CAD build for the part. Positions are in the model's coordinates, mm. A direction names the side the tool comes from. Round coordinates to 2 decimals unless told otherwise and drop trailing zeros. Loops run counter-clockwise (first coordinate to the right, second up) from the corner with the lowest first, then second, coordinate; pieces in that order, holes last.
from build123d import *

# Parameters (mm, degrees)
F1_DEPTH = 12.7
F2_R     = 6.35
F3_DEPTH = 76.201
F4_R     = 6.35
F5_DEPTH = 12.7


with BuildPart() as f1:
    # F0 (on Top) → F1 (new body, symmetric)
    with BuildSketch(Plane.XY):
        Polygon((12.7, -38.1), (12.7, 0), (12.7, 38.1), (-12.7, 38.1), (-12.7, 12.7), (-38.1, 12.7), (-38.1, 0), (-38.1, -12.7), (-12.7, -12.7), (-12.7, -38.1), align=None)
    extrude(amount=F1_DEPTH, both=True)

    # F2 (on face) → F3 (cut, through all)
    with BuildSketch(Plane(origin=(0, 38.1, 0), x_dir=(-1, 0, 0), z_dir=(0, 1, 0))):
        Circle(F2_R)
    extrude(amount=-F3_DEPTH, mode=Mode.SUBTRACT)

    # F4 (on face) → F5 (cut)
    with BuildSketch(Plane(origin=(-38.1, 0, 0), x_dir=(0, -1, 0), z_dir=(-1, 0, 0))):
        Circle(F4_R)
    extrude(amount=-F5_DEPTH, mode=Mode.SUBTRACT)


solid = f1.part
Item 1: Cut at C-C (y = 0). List the corners of the cut face in (x, z), plus the area to 3 significant figures.
Verdict:
outline: (-38.1, -12.7) - (12.7, -12.7) - (12.7, 12.7) - (-38.1, 12.7) - (-38.1, 6.35) - (-25.4, 6.35) - (-25.4, -6.35) - (-38.1, -6.35) - close; hole circle Ø12.7 at (0, 0)
area: 1,000 mm2
Item 2: Mould opens along Y. For faces 4 (the cylindrical face through (1.38, 0.53, -6.2)), 5 (the flat face through (3, 38.1, 6)), 6 (the flat face through (-25.4, 0, 0)) say: released by +Y, released by -Y, zero draft, split by the parting line, or undercut.
Verdict:
face 4: zero draft
face 5: released by +Y
face 6: undercut
Item 3: Wall check: L1, parallel to Z at x = -31.5, y = 0; L2, parallel to X at y = -28, z = -9.25; L3, parallel to X at y = 30.5, z = -3.25. Give the ranges that are in metal, low to high.
Verdict:
L1: z = -12.7 to -6.35, 6.35 to 12.7
L2: x = -12.7 to 12.7
L3: x = -12.7 to -5.46, 5.46 to 12.7
Item 4: 3-axis set-ups, long thin cutter, end or side, ignore diameter. For faces 1 (the flat face through (-26, -12.7, 0)), 2 (the cylindrical face through (-31.84, 1.38, -6.2)), 3 (the flat face through (-12.7, 26, 0)): which of +Z, -Z, +X, -X, +Y, -Y reach the whole face in a straight line?
Verdict:
face 1: +Z, -Z, -X, -Y
face 2: -X
face 3: +Z, -Z, -X, +Y
Item 5: Cut at D-D (z = 0). List the corners of the cut face in (x, y), plus the area to 3 significant figures.
Verdict:
outline: (-38.1, -12.7) - (-12.7, -12.7) - (-12.7, -38.1) - (-6.35, -38.1) - (-6.35, 38.1) - (-12.7, 38.1) - (-12.7, 12.7) - (-38.1, 12.7) - (-38.1, 6.35) - (-25.4, 6.35) - (-25.4, -6.35) - (-38.1, -6.35) - close; (6.35, -38.1) - (12.7, -38.1) - (12.7, 38.1) - (6.35, 38.1) - close
area: 1,450 mm2
Item 6: Flat gauge pins, fed straight in: P1, Ø4, axis at y = -16.5, z = 4.5, coming from the -X side; P2, Ø8, axis at x = -23.5, z = -3.5, coming from the +Y side; P3, Ø7.5, axis at x = -26.5, z = -3, coming from the -Y side. Where does each tip first touch, or does it go through?
Verdict:
P1: stops at x = -12.7
P2: stops at y = 12.7
P3: stops at y = -12.7
Item 7: Cut at A-A (x = 0). List the corners of the cut face in (y, z), plus the area to 3 significant figures.
Verdict:
outline: (-38.1, -12.7) - (38.1, -12.7) - (38.1, -6.35) - (-38.1, -6.35) - close; (-38.1, 6.35) - (38.1, 6.35) - (38.1, 12.7) - (-38.1, 12.7) - close
area: 968 mm2
Item 8: Cut at B-B (z = 9.5). List the corners of the cut face in (x, y), plus the area to 3 significant figures.
Verdict:
outline: (-38.1, -12.7) - (-12.7, -12.7) - (-12.7, -38.1) - (12.7, -38.1) - (12.7, 38.1) - (-12.7, 38.1) - (-12.7, 12.7) - (-38.1, 12.7) - close
area: 2,580 mm2
